Could you check a few things on this model? Use its own coordinates, in mm. Face numbers are marked on the shaded views. Give positions to 0.01 mm unless a question says otherwise; leave off trailing zeros. Order: outer loops, then holes, each group sorted by start corner. A loop starts at its lowest first (then second) coordinate and runs counter-clockwise, first axis right, second up. Notation, with made-up numbers: M 28.25,79.5 L 54.25,79.5 A19 ccw 54.25,107.5 Z; hole C -31.5,-9 d11. An arc over 180 degrees is marked long. Use a Markdown table: item, result. Add a question column.
Item 1: Suppose I cut it at A-A on z = -60. Write out the boundary of the cut face in (x, y).
Item 2: Suppose I cut it at C-C on z = -16. Write out the boundary of the cut face in (x, y), plus the area to 3 significant figures.
Item 3: I'm going to push flat-ended pins straight in: pin 1 Ø1.6 at (y, z) = (-1, 6.5) entering from +X; pin 2 Ø1.1 at (y, z) = (3, -27) entering from +X; pin 3 Ø1 at (x, y) = (31.5, 0.5) entering from +Z. Where does each tip first touch, or does it pass through?
Item 4: If we mould it in two halves opening along Z, with no side actions, what happens to the marked faces 1 and 2? For each: released by +Z, released by -Z, zero draft, split by the parting line, or undercut.
Item 5: Suppose I cut it at B-B on x = 32.5. Write out the boundary of the cut face in (y, z), plus the area to 3 significant figures.
Item 6: If I drill on L1, parallel to Z at x = 3.5, y = 0.25; L2, parallel to X at y = 4.75, z = -16; L3, parallel to Y at x = 33, z = -35, over which ranges is the centre line in solid material (lowest first)? Write a range as from..to.
Item 7: Suppose I cut it at D-D on y = 3.75. Write out the boundary of the cut face in (x, z).
from build123d import *

# Parameters (mm, degrees)
SKETCH1_W           = 37
SKETCH1_H           = 62
SKETCH1_R           = 1.15
BOSS_EXTRUDE1_DEPTH = 1.2
SKETCH2_W           = 36
SKETCH2_H           = 53
BOSS_EXTRUDE2_DEPTH = 3.7
SKETCH3_R           = 0.75
CUT_EXTRUDE1_DEPTH  = 73.295850503
SKETCH4_R           = 5
SKETCH4_R_2         = 1.786053174
BOSS_EXTRUDE3_DEPTH = 0.1
SKETCH5_W           = 20.937122204
SKETCH5_H           = 23.749430493
BOSS_EXTRUDE4_DEPTH = 2


with BuildPart() as part:
    # Sketch1 → Boss-Extrude1 (new body)
    with BuildSketch(Plane(origin=(0, 0, 0), x_dir=(1, 0, 0), z_dir=(0, 1, 0))):
        with Locations((18.5, 31)):
            Rectangle(SKETCH1_W, SKETCH1_H)
        with Locations(Location((32.5, 60, 0), (0, 0, 270))):
            Circle(SKETCH1_R, mode=Mode.SUBTRACT)
        with Locations(Location((4.5, 60, 0), (0, 0, 270))):
            Circle(SKETCH1_R, mode=Mode.SUBTRACT)
        with Locations(Location((32.5, 2, 0), (0, 0, 270))):
            Circle(SKETCH1_R, mode=Mode.SUBTRACT)
        with Locations(Location((4.5, 2, 0), (0, 0, 270))):
            Circle(SKETCH1_R, mode=Mode.SUBTRACT)
    extrude(amount=BOSS_EXTRUDE1_DEPTH)

    # Sketch2 → Boss-Extrude2 (add)
    with BuildSketch(Plane(origin=(0, 1.2, 0), x_dir=(1, 0, 0), z_dir=(0, 1, 0))):
        with Locations((18.5, 31)):
            Rectangle(SKETCH2_W, SKETCH2_H)
    extrude(amount=BOSS_EXTRUDE2_DEPTH)

    # Sketch3 → Cut-Extrude1 (cut, through all)
    with BuildSketch(Plane(origin=(0, 1.2, 0), x_dir=(1, 0, 0), z_dir=(0, 1, 0))):
        with Locations(Location((9.031578358, 2.050688375, 0), (0, 0, 270))):
            Circle(SKETCH3_R)
        with Locations(Location((11.531578358, 2.050688375, 0), (0, 0, 270))):
            Circle(SKETCH3_R)
        with Locations(Location((14.031578358, 2.050688375, 0), (0, 0, 270))):
            Circle(SKETCH3_R)
        with Locations(Location((16.531578358, 2.050688375, 0), (0, 0, 270))):
            Circle(SKETCH3_R)
        with Locations(Location((19.031578358, 2.050688375, 0), (0, 0, 270))):
            Circle(SKETCH3_R)
        with Locations(Location((21.531578358, 2.050688375, 0), (0, 0, 270))):
            Circle(SKETCH3_R)
        with Locations(Location((24.031578358, 2.050688375, 0), (0, 0, 270))):
            Circle(SKETCH3_R)
        with Locations(Location((26.531578358, 2.050688375, 0), (0, 0, 270))):
            Circle(SKETCH3_R)
    extrude(amount=-CUT_EXTRUDE1_DEPTH, mode=Mode.SUBTRACT)

    # Sketch4 → Boss-Extrude3 (add)
    # profile 1 of 3: a face of its own
    with BuildSketch(Plane(origin=(0, 4.9, 0), x_dir=(1, 0, 0), z_dir=(0, 1, 0))):
        with Locations(Location((26.639884222, 48.5, 0), (0, 0, 270))):
            Circle(SKETCH4_R)
        with Locations(Location((24.763300075, 48.058155317, 0), (0, 0, 270))):
            Circle(SKETCH4_R_2, mode=Mode.SUBTRACT)
    # profile 2 of 3: a face of its own
    with BuildSketch(Plane(origin=(0, 4.9, 0), x_dir=(1, 0, 0), z_dir=(0, 1, 0))):
        with Locations(Location((26.639884222, 13.5, 0), (0, 0, 270))):
            Circle(SKETCH4_R)
        with Locations(Location((24.763300075, 12.971685579, 0), (0, 0, 270))):
            Circle(SKETCH4_R_2, mode=Mode.SUBTRACT)
    # profile 3 of 3: a face of its own
    with BuildSketch(Plane(origin=(0, 4.9, 0), x_dir=(1, 0, 0), z_dir=(0, 1, 0))):
        with BuildLine():
            ThreePointArc((11.640146641, 47.414213562), (4.841156768, 31), (11.640146641, 14.585786438))
            ThreePointArc((11.640146641, 14.585786438), (14.468573766, 14.585786438), (14.468573766, 17.414213562))
            ThreePointArc((14.468573766, 17.414213562), (8.841156768, 31), (14.468573766, 44.585786438))
            ThreePointArc((14.468573766, 44.585786438), (14.468573766, 47.414213562), (11.640146641, 47.414213562))
        make_face()
    extrude(amount=BOSS_EXTRUDE3_DEPTH)

    # Sketch5 → Boss-Extrude4 (add)
    with BuildSketch(Plane.XZ):
        with Locations((17.860565838, 7.383650804)):
            Rectangle(SKETCH5_W, SKETCH5_H)
    extrude(amount=BOSS_EXTRUDE4_DEPTH)


solid = part.part
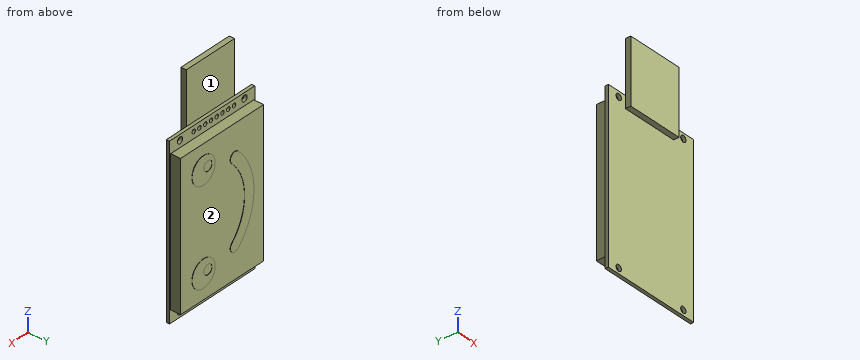
Findings below:
| question | item | result |
|---|---|---|
| 1 | outline | M 0,0 L 3.35,0 L 3.35,1.2 L 0,1.2 Z; M 5.65,0 L 31.35,0 L 31.35,1.2 L 5.65,1.2 Z; M 33.65,0 L 37,0 L 37,1.2 L 33.65,1.2 Z |
| 2 | outline | M 0,0 L 37,0 L 37,1.2 L 36.5,1.2 L 36.5,4.9 L 30.97,4.9 L 30.97,5 L 22.31,5 L 22.31,4.9 L 15.05,4.9 L 15.05,5 L 10.34,5 L 10.34,4.9 L 0.5,4.9 L 0.5,1.2 L 0,1.2 Z |
| 2 | area | 179 mm^2 |
| 3 | pin 1 | stops at x = 28.33 |
| 3 | pin 2 | stops at x = 36.5 |
| 3 | pin 3 | stops at z = 0 |
| 4 | face 1 | zero draft |
| 4 | face 2 | undercut |
| 5 | outline | M 0,-62 L 1.2,-62 L 1.2,-61.15 L 0,-61.15 Z; M 0,-58.85 L 1.2,-58.85 L 1.2,-57.5 L 4.9,-57.5 L 4.9,-4.5 L 1.2,-4.5 L 1.2,-3.15 L 0,-3.15 Z; M 0,-0.85 L 1.2,-0.85 L 1.2,0 L 0,0 Z |
| 5 | area | 265 mm^2 |
| 6 | L1 | z = -62..-60.57, -59.43..-2.57, -1.43..0 |
| 6 | L2 | x = 0.5..36.5 |
| 6 | L3 | y = 0..4.9 |
| 7 | outline | M 0.5,-57.5 L 36.5,-57.5 L 36.5,-4.5 L 0.5,-4.5 Z |
